Can you work these out from the model? Positions are in its coordinate system, mm. Coordinates: 2 decimals unless noted, no trailing zeros. Write each loop counter-clockwise with the first axis right and the second up, starting at its lowest first coordinate (ties: lowest second). Pieces come first, ordered by that corner, then holes. Notation, with made-up numbers: M -34.75,-7.5 L -19.75,-7.5 A20 cw -19.75,21.5 Z; hole C 73.25,11.25 d7. An arc over 180 degrees is marked long. Answer as a JSON object with one key per item and string values. Group by question number.
from build123d import *

# Parameters (mm, degrees)
SKETCH2_W          = 728.6625
SKETCH2_H          = 238.125
EXTRUDE1_DEPTH     = 17.78
SKETCH3_R          = 1.5875
SKETCH3_R_2        = 3.175
SKETCH3_W          = 25.4
SKETCH3_H          = 50.8
CUT_EXTRUDE1_DEPTH = 17.78
SKETCH6_R          = 3.302
CUT_EXTRUDE4_DEPTH = 17.78
SKETCH4_W          = 169.8625
SKETCH4_H          = 8.255
CUT_EXTRUDE2_DEPTH = 3.175
CUT_EXTRUDE3_DEPTH = 5.08
SKETCH7_R          = 3.302
CUT_EXTRUDE5_DEPTH = 5.08
SKETCH8_R          = 4.7625
CUT_EXTRUDE6_DEPTH = 17.78


with BuildPart() as part:
    # Sketch2 → Extrude1 (new body)
    with BuildSketch(Plane.XY):
        with Locations((-5376.06875, 779.4625)):
            Rectangle(SKETCH2_W, SKETCH2_H)
    extrude(amount=-EXTRUDE1_DEPTH)

    # Sketch3 → Cut-Extrude1 (cut)
    with BuildSketch(Plane.XY):
        with Locations((-5702.3, 892.175)):
            Circle(SKETCH3_R)
        with Locations((-5734.05, 860.425)):
            Circle(SKETCH3_R)
        with Locations((-5734.05, 698.5)):
            Circle(SKETCH3_R)
        with Locations((-5702.3, 666.75)):
            Circle(SKETCH3_R)
        with Locations((-5569.74375, 684.2125)):
            Circle(SKETCH3_R_2)
        with Locations((-5512.59375, 684.2125)):
            Circle(SKETCH3_R_2)
        with Locations((-5474.890625, 666.75)):
            Circle(SKETCH3_R)
        with Locations((-5277.246875, 666.75)):
            Circle(SKETCH3_R)
        with Locations((-5239.54375, 684.2125)):
            Circle(SKETCH3_R_2)
        with Locations((-5182.39375, 684.2125)):
            Circle(SKETCH3_R_2)
        with Locations((-5049.8375, 666.75)):
            Circle(SKETCH3_R)
        with Locations((-5018.0875, 698.5)):
            Circle(SKETCH3_R)
        with Locations((-5018.0875, 860.425)):
            Circle(SKETCH3_R)
        with Locations((-5049.8375, 892.175)):
            Circle(SKETCH3_R)
        with Locations((-5277.246875, 892.175)):
            Circle(SKETCH3_R)
        with Locations((-5474.890625, 892.175)):
            Circle(SKETCH3_R)
        with Locations((-5278.4375, 777.875)):
            Rectangle(SKETCH3_W, SKETCH3_H)
    extrude(amount=-CUT_EXTRUDE1_DEPTH, mode=Mode.SUBTRACT)

    # Sketch6 → Cut-Extrude4 (cut)
    with BuildSketch(Plane.XY):
        with Locations((-5288.802633409, 800.940133409)):
            Circle(SKETCH6_R)
        with Locations((-5268.072366591, 800.940133409)):
            Circle(SKETCH6_R)
        with Locations((-5288.802633409, 754.809866591)):
            Circle(SKETCH6_R)
        with Locations((-5268.072366591, 754.809866591)):
            Circle(SKETCH6_R)
    extrude(amount=-CUT_EXTRUDE4_DEPTH, mode=Mode.SUBTRACT)

    # Sketch4 → Cut-Extrude2 (cut)
    with BuildSketch(Plane.XZ.offset(-660.4)):
        with Locations((-5376.06875, -13.6525)):
            Rectangle(SKETCH4_W, SKETCH4_H)
    extrude(amount=-CUT_EXTRUDE2_DEPTH, mode=Mode.SUBTRACT)

    # Sketch5 → Cut-Extrude3 (cut)
    with BuildSketch(Plane(origin=(0, 0, -17.78), x_dir=(-1, 0, 0), z_dir=(0, 0, -1))):
        Polygon((5011.7375, 660.4), (5113.3375, 660.4), (5113.3375, 673.1), (5024.4375, 673.1), (5024.4375, 885.825), (5727.7, 885.825), (5727.7, 673.1), (5638.8, 673.1), (5638.8, 660.4), (5740.4, 660.4), (5740.4, 898.525), (5011.7375, 898.525), align=None)
    extrude(amount=-CUT_EXTRUDE3_DEPTH, mode=Mode.SUBTRACT)

    # Sketch7 → Cut-Extrude5 (cut)
    with BuildSketch(Plane(origin=(0, 0, -17.78), x_dir=(-1, 0, 0), z_dir=(0, 0, -1))):
        with Locations((5641.525003649, 671.235178531)):
            Circle(SKETCH7_R)
        with Locations((5110.612496351, 671.235178531)):
            Circle(SKETCH7_R)
    extrude(amount=-CUT_EXTRUDE5_DEPTH, mode=Mode.SUBTRACT)

    # Sketch8 → Cut-Extrude6 (cut)
    with BuildSketch(Plane(origin=(0, 0, -17.78), x_dir=(-1, 0, 0), z_dir=(0, 0, -1))):
        with Locations((5713.73, 835.025)):
            Circle(SKETCH8_R)
        with Locations((5712.46, 819.785)):
            Circle(SKETCH8_R)
        with Locations((5712.46, 802.005)):
            Circle(SKETCH8_R)
        with Locations((5712.46, 784.225)):
            Circle(SKETCH8_R)
    extrude(amount=-CUT_EXTRUDE6_DEPTH, mode=Mode.SUBTRACT)


solid = part.part
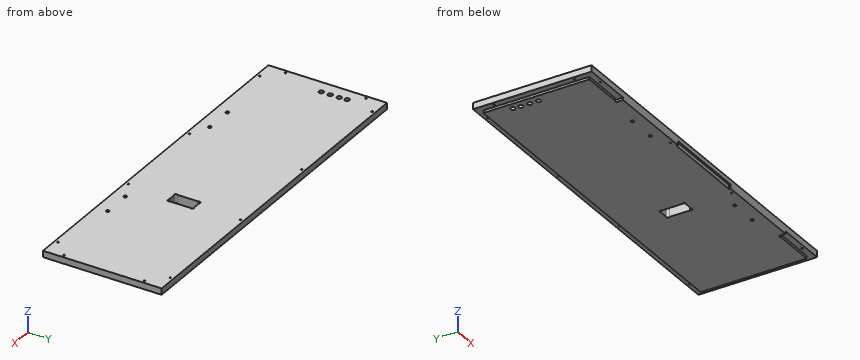
Q1. Will these pins go through, and if not, where does the flat tip stop? pin 1 (4 mm diameter, centred on x = -5569.74, y = 684.21, fed in from -Z); pin 2 (1.5 mm diameter, centred on x = -5705.5, z = -15.5, fed in from -Y); pin 3 (2.5 mm diameter, centred on y = 778, z = -16, fed in from -X); pin 4 (1.6 mm diameter, centred on y = 662.5, z = -14, fed in from +X).
Q2. If we section it at A-A on x = -5172: List the corners of the cut face in (y, z) for me (3 decimals).
Q3. Please list where these lines run through material, in increasing order: L1, parallel to X at y = 769, z = -12; L2, parallel to X at y = 788, z = -9.5; L3, parallel to Y at x = -5713.73, z = -8 (1 decimal).
Q4. If we section it at B-B on x = -5350.5: List the corners of the cut face in (y, z) for me (3 decimals).
Reply:
{
 "1": {"pin 1": "through", "pin 2": "y = 673.1", "pin 3": "x = -5727.7", "pin 4": "x = -5113.34"},
 "2": {"outline": "M 660.4,-17.78 L 885.825,-17.78 L 885.825,-12.7 L 898.525,-12.7 L 898.525,0 L 660.4,0 Z"},
 "3": {"L1": "-5740.4 to -5291.14, -5265.74 to -5011.74", "L2": "-5740.4 to -5715.36, -5709.56 to -5291.14, -5265.74 to -5011.74", "L3": "660.4 to 779.6, 788.8 to 797.4, 806.6 to 815.2, 824.4 to 830.3, 839.8 to 898.5"},
 "4": {"outline": "M 660.4,-9.525 L 663.575,-9.525 L 663.575,-17.78 L 885.825,-17.78 L 885.825,-12.7 L 898.525,-12.7 L 898.525,0 L 660.4,0 Z"}
}
